Input: part model. Units: mm. Frame: model coordinates. Face numbers are marked on the shaded views. A direction names the side the tool comes from. Give positions to 0.01 mm unless a question says otherwise; leave off trailing zeros. Loops run counter-clockwise (first coordinate to the right, second up) from the corner with the lowest first, then second, coordinate; pieces in that order, holes last. Notation, with made-up numbers: (38.25, 15) - (64.25, 15) arc R30 ccw to (64.25, 43) - close; hole circle Ø1 at (72, -20). An arc over 180 degrees is marked (long way). One line per item, written item: value.
from build123d import *

# Parameters (mm, degrees)
F0_W     = 50.8
F0_H     = 38.1
F1_DEPTH = 31.75
F2_R     = 25.4
F3_DEPTH = 50.801
F4_W     = 25.4
F4_H     = 19.05
F5_DEPTH = 31.751


with BuildPart() as f1:
    # F0 (on Front) → F1 (new body)
    with BuildSketch(Plane.XZ):
        with Locations((25.4, 19.05)):
            Rectangle(F0_W, F0_H)
    extrude(amount=F1_DEPTH)

    # F2 (on Right) → F3 (cut, through all)
    with BuildSketch(Plane.YZ):
        with Locations((-31.75, 37.877075)):
            Circle(F2_R)
    extrude(amount=F3_DEPTH, mode=Mode.SUBTRACT)

    # F4 (on Front) → F5 (cut, through all)
    with BuildSketch(Plane.XZ):
        with Locations((25.4, 28.575)):
            Rectangle(F4_W, F4_H)
    extrude(amount=F5_DEPTH, mode=Mode.SUBTRACT)


solid = f1.part
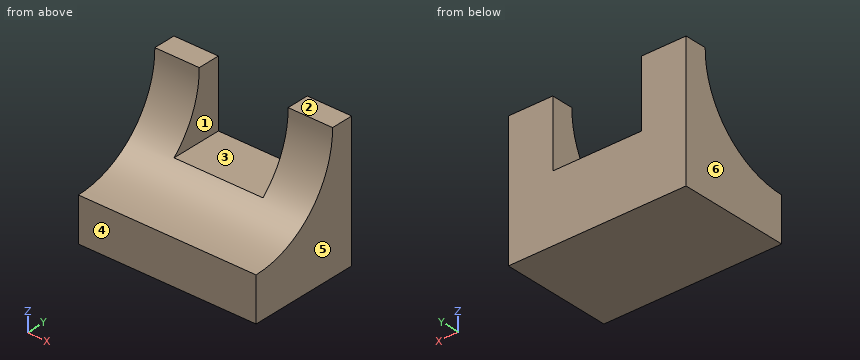
Item 1: Draft query along X for the marked faces 3, 4, 5 and 6. Return one class per face: pulls with the +X half, pulls with the -X half, needs draft (parallel to the pull), parting line crosses it, or undercut.
Verdict:
face 3: undercut
face 4: needs draft
face 5: pulls with the +X half
face 6: pulls with the -X half
Item 2: Access query for the marked faces 1 and 2. Directions: +Z, -Z, +X, -X, +Y, -Y. A direction counts if a zero-diameter tool reaches every point of the face in a straight line with its end or side. Return the directions, or none.
Verdict:
face 1: +Z, +Y, -Y
face 2: +Z, +X, -X, +Y, -Y
Item 3: Section D-D, the plane z = 25. Output: boundary loops of the cut face in (x, y), and give its area (3 significant figures).
Verdict:
outline: (0, -9.86) - (12.7, -9.86) - (12.7, 0) - (0, 0) - close; (38.1, -9.86) - (50.8, -9.86) - (50.8, 0) - (38.1, 0) - close
area: 250 mm^2
Item 4: Section A-A, the plane z = 33.5. Output: boundary loops of the cut face in (x, y).
Verdict:
outline: (0, -6.73) - (12.7, -6.73) - (12.7, 0) - (0, 0) - close; (38.1, -6.73) - (50.8, -6.73) - (50.8, 0) - (38.1, 0) - close
Item 5: Section C-C, the plane y = -14. Output: boundary loops of the cut face in (x, z).
Verdict:
outline: (0, 0) - (50.8, 0) - (50.8, 19.71) - (38.1, 19.71) - (38.1, 19.05) - (12.7, 19.05) - (12.7, 19.71) - (0, 19.71) - close
Item 6: Pin query (flat end, axial travel): P1, Ø6, axis at x = 25.5, y = -26, coming from the +Z side; P2, Ø5, axis at x = 27, y = -5, coming from the +Z side; P3, Ø1.5, axis at x = 8, y = -19.5, coming from the +Z side; P4, Ø4.5, axis at y = -11, z = 33, coming from the -X side. Return the tip coordinate at first contact, or that it passes through.
Verdict:
P1: stops at z = 14.03
P2: stops at z = 19.05
P3: stops at z = 16.06
P4: passes through
Item 7: Material intervals for L1, parallel to Z at x = 19, y = -8.5; L2, parallel to Z at x = 23, y = -26; L3, parallel to Y at x = 4.5, z = 29.5, sorted ascending.
Verdict:
L1: z = 0 to 19.05
L2: z = 0 to 13.14
L3: y = -7.77 to 0
Item 8: Section B-B, the plane x = 20. Output: boundary loops of the cut face in (y, z), and give its area (3 significant figures).
Verdict:
outline: (-31.75, 0) - (0, 0) - (0, 19.05) - (-14.7, 19.05) arc R25.4 cw to (-31.75, 12.48) - close
area: 528 mm^2
